Read the model definition and answer for the solid it produces. Units are mm, in the model's axes. Round coordinates to 2 decimals unless told otherwise and drop trailing zeros. Write each loop counter-clockwise with the first axis right and the second up, starting at its lowest first coordinate (ties: lowest second). Pieces come first, ordered by that corner, then holes. Notation, with made-up numbers: (17.25, 62.25) - (42.25, 62.25) arc R21 cw to (42.25, 80.25) - close; hole circle Ø6 at (87.5, 24.25). An arc over 180 degrees is marked (long way). Answer as CSV lines item,"result". Start each with the question number.
1) Find section A-A on x = 0. Determine the outline of the cut face in (y, z), then the cut area to 3 significant figures.
2) Find section B-B on z = 0.3. Determine the outline of the cut face in (x, y), then the cut area to 3 significant figures.
3) Consider line 1 along Y through (x, z) = (-22, 1.3); line 2 along Y through (x, z) = (0.5, 1.4); line 3 along Y through (x, z) = (7.5, 1.85). Determine where each line is inside the solid, lowest interval first.
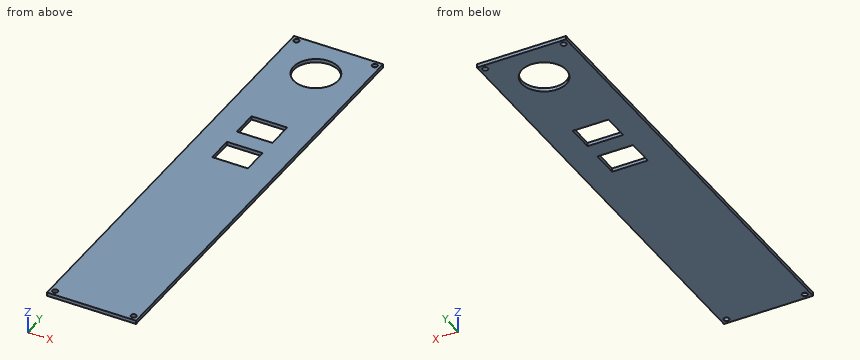
from build123d import *

# Parameters (mm, degrees)
SKETCH1_W           = 50
SKETCH1_H           = 251
BOSS_EXTRUDE1_DEPTH = 2
CUT_EXTRUDE1_REACH  = 130.472
SKETCH2_R           = 12.5
SKETCH6_R           = 1.5
CUT_EXTRUDE5_DEPTH  = 2
SKETCH8_W           = 20
SKETCH8_H           = 15
CUT_EXTRUDE6_DEPTH  = 2


with BuildPart() as part:
    # Sketch1 → Boss-Extrude1 (new body)
    with BuildSketch(Plane(origin=(0, 15.253788563, 0), x_dir=(1, 0, 0), z_dir=(0, 0, 1))):
        with Locations((0, -0.5)):
            Rectangle(SKETCH1_W, SKETCH1_H)
    extrude(amount=BOSS_EXTRUDE1_DEPTH)

    # Sketch2 → Cut-Extrude1 (cut, up to next)
    with BuildSketch(Plane(origin=(0, 15.253788563, 0), x_dir=(-1, 0, 0), z_dir=(0, 0, -1)), mode=Mode.PRIVATE) as cut_extrude1_sk1:
        with Locations((0, 102)):
            Circle(SKETCH2_R)
    cut_extrude1_tool1 = extrude(cut_extrude1_sk1.sketch, amount=-CUT_EXTRUDE1_REACH, mode=Mode.PRIVATE) & part.part
    add(cut_extrude1_tool1.solids().sort_by_distance((0, 117.253789, 0))[0], mode=Mode.SUBTRACT)

    # Sketch6 → Cut-Extrude5 (cut)
    with BuildSketch(Plane(origin=(0, 15.253788563, 2), x_dir=(1, 0, 0), z_dir=(0, 0, 1))):
        with Locations((-22, 122)):
            Circle(SKETCH6_R)
        with Locations((22, 122)):
            Circle(SKETCH6_R)
        with Locations((-22, -123)):
            Circle(SKETCH6_R)
        with Locations((22, -123)):
            Circle(SKETCH6_R)
    extrude(amount=-CUT_EXTRUDE5_DEPTH, mode=Mode.SUBTRACT)

    # Sketch8 → Cut-Extrude6 (cut)
    with BuildSketch(Plane(origin=(0, 0, 0), x_dir=(-1, 0, 0), z_dir=(0, 0, -1))):
        with Locations((0, 62.5)):
            Rectangle(SKETCH8_W, SKETCH8_H)
        with Locations((0, 37.5)):
            Rectangle(SKETCH8_W, SKETCH8_H)
    extrude(amount=-CUT_EXTRUDE6_DEPTH, mode=Mode.SUBTRACT)


solid = part.part
Check values:
1,outline,"(-110.75, 0) - (30, 0) - (30, 2) - (-110.75, 2) - close; (45, 0) - (55, 0) - (55, 2) - (45, 2) - close; (70, 0) - (104.75, 0) - (104.75, 2) - (70, 2) - close; (129.75, 0) - (140.25, 0) - (140.25, 2) - (129.75, 2) - close"
1,area,"392 mm^2"
2,outline,"(-25, -110.75) - (25, -110.75) - (25, 140.25) - (-25, 140.25) - close; hole circle Ø3 at (-22, -107.75); hole circle Ø3 at (-22, 137.25); hole circle Ø25 at (0, 117.25); hole (-10, 30) - (10, 30) - (10, 45) - (-10, 45) - close; hole (-10, 55) - (10, 55) - (10, 70) - (-10, 70) - close; hole circle Ø3 at (22, -107.75); hole circle Ø3 at (22, 137.25)"
2,area,"11,400 mm^2"
3,line 1,"y = -110.75 to -109.25, -106.25 to 135.75, 138.75 to 140.25"
3,line 2,"y = -110.75 to 30, 45 to 55, 70 to 104.76, 129.74 to 140.25"
3,line 3,"y = -110.75 to 30, 45 to 55, 70 to 107.25, 127.25 to 140.25"
